```python
from build123d import *

# Parameters (mm, degrees)
BOSS_EXTRUDE1_DEPTH          = 36
SKETCH2_R                    = 15
CUT_EXTRUDE1_DEPTH           = 1
SKETCH3_R                    = 10
SKETCH3_R_2                  = 5
BOSS_EXTRUDE2_DEPTH          = 2
BOSS_EXTRUDE3_DEPTH          = 32
F_3_0_3_DIAMETER_HOLE1_D     = 3
F_3_0_3_DIAMETER_HOLE1_DEPTH = 5
F_3_0_3_DIAMETER_HOLE1_TIP   = 0.901290929
SKETCH7_W                    = 20
SKETCH7_H                    = 3
BOSS_EXTRUDE4_DEPTH          = 10


with BuildPart() as part:
    # Sketch1 → Boss-Extrude1 (new body)
    with BuildSketch(Plane(origin=(0, 0, 0), x_dir=(1, 0, 0), z_dir=(0, 1, 0))):
        Polygon((-20.5, 18.5), (-18.5, 20.5), (18.5, 20.5), (20.5, 18.5), (20.5, -18.5), (18.5, -20.5), (-18.5, -20.5), (-20.5, -18.5), align=None)
    extrude(amount=BOSS_EXTRUDE1_DEPTH)

    # Sketch2 → Cut-Extrude1 (cut)
    with BuildSketch(Plane(origin=(0, 36, 0), x_dir=(-1, 0, 0), z_dir=(0, 1, 0))):
        with Locations(Location((0, 0, 0), (0, 0, 90))):
            Circle(SKETCH2_R)
    extrude(amount=-CUT_EXTRUDE1_DEPTH, mode=Mode.SUBTRACT)

    # Sketch3 → Boss-Extrude2 (add)
    with BuildSketch(Plane(origin=(0, 35, 0), x_dir=(1, 0, 0), z_dir=(0, 1, 0))):
        with Locations(Location((0, 0, 0), (0, 0, 270))):
            Circle(SKETCH3_R)
        with Locations(Location((0, 0, 0), (0, 0, 270))):
            Circle(SKETCH3_R_2, mode=Mode.SUBTRACT)
    extrude(amount=BOSS_EXTRUDE2_DEPTH)

    # Sketch4 → Boss-Extrude3 (add)
    with BuildSketch(Plane(origin=(0, 35, 0), x_dir=(1, 0, 0), z_dir=(0, 1, 0))):
        with BuildLine():
            Line((-1.470984161, 2.175359116), (1.470984161, 2.175359116))
            ThreePointArc((1.470984161, 2.175359116), (0, -2.626020123), (-1.470984161, 2.175359116))
        make_face()
    extrude(amount=BOSS_EXTRUDE3_DEPTH)

    # 3.0 _3_ Diameter Hole1
    with Locations(Plane(origin=(0, 36, 0), x_dir=(-1, 0, 0), z_dir=(0, 1, 0))):
        with Locations((-15.5, -15.5), (15.5, -15.5), (15.5, 15.5), (-15.5, 15.5)):
            Hole(F_3_0_3_DIAMETER_HOLE1_D / 2, depth=F_3_0_3_DIAMETER_HOLE1_DEPTH)
            with Locations((0, 0, -(F_3_0_3_DIAMETER_HOLE1_DEPTH + F_3_0_3_DIAMETER_HOLE1_TIP / 2))):  # 118° drill point
                Cone(0, F_3_0_3_DIAMETER_HOLE1_D / 2, F_3_0_3_DIAMETER_HOLE1_TIP, mode=Mode.SUBTRACT)

    # Sketch7 → Boss-Extrude4 (add)
    with BuildSketch(Plane(origin=(0, 0, -20.5), x_dir=(-1, 0, 0), z_dir=(0, 0, -1))):
        with Locations((-0.141546157, 1.5)):
            Rectangle(SKETCH7_W, SKETCH7_H)
    extrude(amount=BOSS_EXTRUDE4_DEPTH)


solid = part.part
```
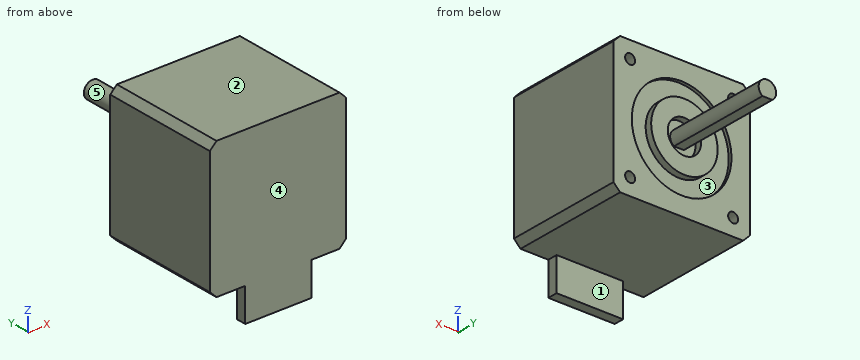
Verification items for the finished model (mm, model axes). Face numbers are marked on the shaded views. A direction names the side the tool comes from. Coordinates: 2 decimals unless noted, no trailing zeros. Loops run counter-clockwise (first coordinate to the right, second up) from the corner with the lowest first, then second, coordinate; pieces in that order, holes last. Notation, with made-up numbers: (-15, 85) - (39, 85) arc R33 ccw to (39, 117) - close; hole circle Ø6 at (-37, 67). An arc over 180 degrees is marked (long way). Answer as a JSON object with one key per item and string values.
(1) Cross-section at D-D, the plane y = 58.5. Record the boundary of the cut face in (x, z).
Response:
{"outline": "(-1.47, -2.18) - (1.47, -2.18) arc R2.63 ccw (long way) to start"}
(2) Scan lines: line 1 along X through (y, z) = (32.2, -15.5); line 2 along X through (y, z) = (35.55, 0). Record each from-to range of solid material in increasing order.
Response:
{"line 1": "x = -20.5 to -17, -14 to 14, 17 to 20.5", "line 2": "x = -20.5 to -15, -10 to -5, -2.63 to 2.63, 5 to 10, 15 to 20.5"}
(3) Go/stop test with flat-tipped pins: pin 1 Ø2.5 at (x, y) = (0.5, 51) entering from -Z; pin 2 Ø1.8 at (x, z) = (-15.5, 15.5) entering from +Y; pin 3 Ø1.5 at (y, z) = (1.5, -28) entering from +X. Record where each tip stops, or that it passes through.
Response:
{"pin 1": "stops at z = -2.18", "pin 2": "stops at y = 30.64", "pin 3": "stops at x = 10.14"}
(4) Mould release check, pull along Z, two halves, no side actions. Record for the marked faces 1, 2 and 3: pulls with the +Z half, pulls with the -Z half, needs draft (parallel to the pull), parting line crosses it, or undercut.
Response:
{"face 1": "needs draft", "face 2": "pulls with the +Z half", "face 3": "undercut"}
(5) Cross-section at C-C, the plane z = 0. Record the boundary of the cut face in (x, y).
Response:
{"outline": "(-20.5, 0) - (20.5, 0) - (20.5, 36) - (15, 36) - (15, 35) - (10, 35) - (10, 37) - (5, 37) - (5, 35) - (2.63, 35) - (2.63, 67) - (-2.63, 67) - (-2.63, 35) - (-5, 35) - (-5, 37) - (-10, 37) - (-10, 35) - (-15, 35) - (-15, 36) - (-20.5, 36) - close"}
(6) Cross-section at A-A, the plane z = -12. Record the boundary of the cut face in (x, y).
Response:
{"outline": "(-20.5, 0) - (20.5, 0) - (20.5, 36) - (9, 36) - (9, 35) - (-9, 35) - (-9, 36) - (-20.5, 36) - close"}
(7) Cross-section at B-B, the plane y = 13. Record the boundary of the cut face in (x, z).
Response:
{"outline": "(-20.5, -18.5) - (-18.5, -20.5) - (18.5, -20.5) - (20.5, -18.5) - (20.5, 18.5) - (18.5, 20.5) - (-18.5, 20.5) - (-20.5, 18.5) - close"}
(8) Access from +Z, -Z, +X, -X, +Y, -Y to the whole of each face (thin tool, end or side, straight path). Record for the marked faces 4 and 5.
Response:
{"face 4": "+Z, -Z, +X, -X, -Y", "face 5": "+Y"}
